The listing builds one solid part. Answer for the finished solid, in the listing's coordinates (mm). Face numbers are marked on the shaded views. Give positions to 0.01 mm unless a question says otherwise; leave off trailing zeros. Order: outer loops, then holes, each group sorted by start corner. A loop starts at its lowest first (then second) coordinate and runs counter-clockwise, first axis right, second up. Notation, with made-up numbers: (-10.5, -30) - (19.5, -30) arc R9 ccw to (19.5, -14) - close; hole circle Ø4 at (-24, 80). An arc over 180 degrees is marked (long way). Use a Markdown table: item, result. Add a question column.
1) Flat-ended cylindrical pins translate along their axes: pin 1 (3 mm diameter, centred on y = 17, z = -10.5, fed in from +X); pin 2 (6 mm diameter, centred on y = -11, z = -5.5, fed in from -X); pin 3 (1.5 mm diameter, centred on y = 10, z = 24.5, fed in from -X); pin 4 (5 mm diameter, centred on x = -25, y = -19, fed in from +Z). Find the tip coordinate at first contact, or state that the pin passes through.
2) Straight lines are drawn through the part: line 1 (Y direction, x = -18, z = 0); line 2 (Z direction, x = -36, y = 5.5); line 3 (X direction, y = 27, z = -10). For each, find the intervals that lie inside material, in ascending order.
3) Find section A-A, the plane y = 0. Determine the outline of the cut face in (x, z).
4) The mould has two halves that part along Y. Classify the marked faces 1, 2 and 3: released by +Y, released by -Y, zero draft, split by the parting line, or undercut.
5) Find section C-C, the plane x = -49.5. Determine the outline of the cut face in (y, z), plus the area to 3 significant figures.
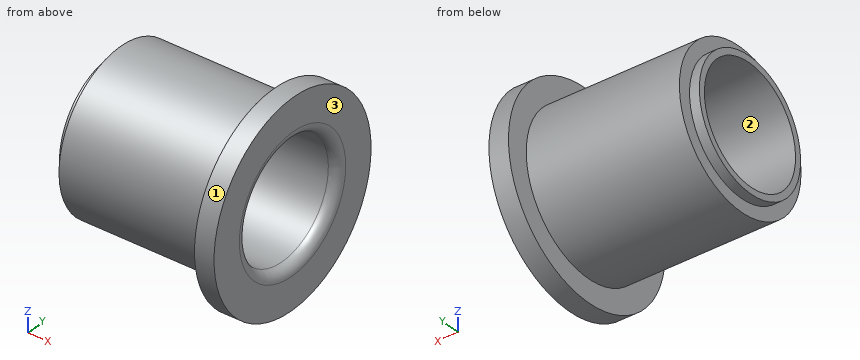
from build123d import *


with BuildPart() as part:
    # Esquisse1 → Base-R_volution (revolve)
    with BuildSketch(Plane.XY, mode=Mode.PRIVATE) as base_r_volution_sk:
        with BuildLine():
            Line((-56, 18), (-3, 18))
            ThreePointArc((-3, 18), (-0.878679656, 18.878679656), (0, 21))
            Line((0, 21), (0, 31))
            Line((0, 31), (-6, 31))
            Line((-6, 31), (-6, 24))
            Line((-6, 24), (-53, 24))
            Line((-53, 24), (-53, 20))
            Line((-53, 20), (-56, 20))
            Line((-56, 20), (-56, 18))
        make_face()
    revolve(base_r_volution_sk.sketch.rotate(Axis((-50.685125628, 0, 0), (1, 0, 0)), 90), axis=Axis((-50.685125628, 0, 0), (1, 0, 0)))


solid = part.part
The answers:
| question | item | result |
|---|---|---|
| 1 | pin 1 | x = 0 |
| 1 | pin 2 | through |
| 1 | pin 3 | x = -6 |
| 1 | pin 4 | z = 17.43 |
| 2 | line 1 | -24 to -18, 18 to 24 |
| 2 | line 2 | -23.36 to -17.14, 17.14 to 23.36 |
| 2 | line 3 | -6 to 0 |
| 3 | outline | (-56, -20) - (-53, -20) - (-53, -24) - (-6, -24) - (-6, -31) - (0, -31) - (0, -21) arc R3 ccw to (-3, -18) - (-56, -18) - close; (-56, 18) - (-3, 18) arc R3 ccw to (0, 21) - (0, 31) - (-6, 31) - (-6, 24) - (-53, 24) - (-53, 20) - (-56, 20) - close |
| 4 | face 1 | split by the parting line |
| 4 | face 2 | undercut |
| 4 | face 3 | zero draft |
| 5 | outline | circle Ø48 at (0, 0); hole circle Ø36 at (0, 0) |
| 5 | area | 792 mm2 |
